Read the model definition and answer for the solid it produces. Units are mm, in the model's axes. Coordinates: 2 decimals unless noted, no trailing zeros. Order: outer loops, then holes, each group sorted by start corner. A loop starts at its lowest first (then second) coordinate and runs counter-clockwise, first axis right, second up.
Autodesk Inventor part; units mm, degrees
ref_plane "YZ Plane" through (0, 0, 0) normal (1, 0, 0) x (0, 1, 0)
ref_plane "XZ Plane" through (0, 0, 0) normal (0, 1, 0) x (-1, 0, 0)
ref_plane "XY Plane" through (0, 0, 0) normal (0, 0, 1) x (1, 0, 0)
sketch "Sketch1" plane through (0, 0, 0) normal (0, 1, 0) x (-1, 0, 0)
  line L0 (25.9, 0) -> (-25.9, 0)
  line L1 (0, -25.9) -> (0, 25.9)
  circle A0 centre (0, 0) radius 18.5 construction
  circle A1 centre (0, 0) radius 13 construction
  dimension "d0" = 37
  dimension "d1" = 26
sketch "Sketch2" plane through (0, 0, 0) normal (0, 1, 0) x (-1, 0, 0)
  line L0 (0, -28.9) -> (0, 26.4)
  line L1 (-60.5, -8) -> (-60.5, -21)
  line L2 (-60.5, -21) -> (60.5, -21)
  line L3 (60.5, -21) -> (60.5, -8)
  line L4 (60.5, -8) -> (-60.5, -8)
  line L5 (-84.7, 0) -> (84.7, 0)
  point P0 (0, 0)
  dimension "d3" = 121
  dimension "d99" = 8
  dimension "d101" = 21
extrude "Extrusion1" add sketch "Sketch2" along normal blind 6
sketch "Sketch6" plane through (0, 0, 0) normal (0, 1, 0) x (-1, 0, 0)
  line L0 (60.5, -21) -> (-60.5, -21)
  line L1 (60.5, -8) -> (60.5, -21)
  line L2 (-60.5, -21) -> (60.5, -21)
  line L3 (60.5, -21) -> (60.5, -8)
  line L4 (-60.5, -8) -> (-60.5, -21)
  line L5 (84.7, 0) -> (-84.7, 0)
  line L6 (0, -28.9) -> (0, 26.4)
  arc A0 (-16, 0) -> (16, 0) centre (0, 0) ccw
  line L7 (16, 0) -> (16, 0)
  line L8 (60.5, 0) -> (-60.5, 0)
  line L9 (16, 0) -> (60.5, 0)
  line L10 (-16, 0) -> (-16, 0)
  line L11 (-16, 0) -> (-60.5, 0)
  point P0 (-17.3617, -21)
  dimension "d18" = 32
extrude "Extrusion5" [suppressed]
sketch "Sketch4" plane through (0, 0, 0) normal (0, 0, 1) x (1, 0, 0)
  line L0 (-18.5, 0) -> (18.5, 0)
  line L1 (18.5, 0) -> (18.5, -2)
  line L2 (18.5, -2) -> (-18.5, -2)
  line L3 (-18.5, -2) -> (-18.5, 0)
  line L4 (-25.9, 0) -> (25.9, 0)
  line L5 (0, -2.4) -> (0, 0.4)
  point P0 (0, 0)
  dimension "d10" = 37
  dimension "d11" = 2
extrude "Extrusion6" [suppressed]
sketch "Sketch5" plane through (0, 0, 0) normal (0, 1, 0) x (-1, 0, 0)
  circle A0 centre (0, 0) radius 18.5 construction
  circle A1 centre (0, 0) radius 18.5 construction
  line L0 (25.9, 0) -> (-25.9, 0)
  line L1 (0, -28.9) -> (0, 26.4)
  line L2 (-18.5, -21) -> (18.5, -21)
  line L3 (18.5, -21) -> (18.5, -18.5)
  line L4 (18.5, -18.5) -> (-18.5, -18.5)
  line L5 (-18.5, -18.5) -> (-18.5, -21)
  dimension "d25" = 37
  dimension "d26" = 21
extrude "Extrusion7" [suppressed]
sketch "Sketch7" plane through (0, 0, 0) normal (0, 0, 1) x (1, 0, 0)
  line L0 (-18.5, 0) -> (18.5, 0)
  line L1 (18.5, 0) -> (18.5, -2)
  line L2 (18.5, -2) -> (-18.5, -2)
  line L3 (-18.5, -2) -> (-18.5, 0)
  line L4 (60.5, 0) -> (-60.5, 0)
  line L5 (-84.7, 0) -> (84.7, 0)
  line L6 (0, -2.4) -> (0, 0.4)
  point P0 (-16, 0)
  point P1 (16, 0)
  dimension "d53" = 2
  dimension "d54" = 18.5
extrude "Extrusion8" [suppressed]
sketch "Sketch8" plane through (0, 0, 0) normal (0, 1, 0) x (-1, 0, 0)
  circle A0 centre (0, 0) radius 12.75
  dimension "d34" = 25.5
extrude "Extrusion9" [suppressed]
pattern_linear "Rectangular Pattern1" [suppressed]
sketch "Sketch9" plane through (0, 6, 0) normal (0, 1, 0) x (1, 0, 0)
  circle A0 centre (0, 0) radius 13
  circle A1 centre (0, 0) radius 15
  dimension "d40" = 26
  dimension "d41" = 30
extrude "Extrusion10" [suppressed]
sketch "Sketch10" plane through (0, 5, 0) normal (0, 1, 0) x (1, 0, 0)
  arc A0 (16, 0) -> (-16, 0) centre (0, 0) ccw
  line L0 (1.5, -18) -> (-1.5, -18)
  line L1 (-29.4, 0) -> (29.4, 0)
  line L2 (0, 36.3) -> (0, -70.8)
  line L3 (1.5, -12) -> (-1.5, -12)
  line L4 (1.5, -12) -> (1.5, -18)
  line L5 (-1.5, -18) -> (-1.5, -12)
  dimension "d48" = 3
  dimension "d49" = 12
  dimension "d50" = 6
extrude "Extrusion11" [suppressed]
fillet "Fillet1" [suppressed]
sketch "Sketch11" plane through (0, 0, 0) normal (0, 1, 0) x (-1, 0, 0)
  line L0 (-60.5, -21) -> (60.5, -21)
  line L1 (60.5, -21) -> (60.5, -47)
  line L2 (60.5, -47) -> (-60.5, -47)
  line L3 (-60.5, -47) -> (-60.5, -21)
  line L4 (84.7, 0) -> (-84.7, 0)
  line L5 (0, -60.1) -> (0, 31.6)
  point P0 (0, 0)
  dimension "d57" = 26
  dimension "d58" = 21
  dimension "d59" = 121
extrude "Extrusion12" add sketch "Sketch11" along normal blind 6
sketch "Sketch12" plane through (0, 0, 0) normal (1, 0, 0) x (0, 1, 0)
  line L0 (6, -8) -> (6, -47)
  arc A0 (6, -16.5081) -> (5.7334, -47) centre (34, -32) ccw
  line L1 (-6.8, 0) -> (40.8, 0)
  line L2 (0, -66) -> (0, 67)
  line L3 (6, -16.5081) -> (6, -47)
  line L4 (6, -47) -> (5.7334, -47)
  line L5 (0, -47) -> (6, -47)
  point P0 (0, 0)
  point P1 (6, 48)
  dimension "d62" = 32
  dimension "d63" = 32
  dimension "d64" = 34
extrude "Extrusion13" cut sketch "Sketch12" along normal through all both and the other way through all
fillet "Fillet3" radius 8 1 edges at (0, 0, -47)
sketch "Sketch13" plane through (0, 0, 0) normal (0, 1, 0) x (-1, 0, 0)
  line L0 (84.7, 0) -> (-84.7, 0)
  line L1 (0, -57.9802) -> (0, 72.5866)
  line L2 (60.5, -8) -> (60.5, -39.3278)
  arc A0 (13.0815, 23.9185) -> (13.0815, 13.0815) centre (18.5, 18.5) ccw
  line L3 (-60.5, -8) -> (-60.5, -16.5081)
  arc A1 (-13.0815, 13.0815) -> (-13.0815, 23.9185) centre (-18.5, 18.5) ccw
  line L4 (18.5, 37) -> (18.5, 0)
  line L5 (-18.5, 0) -> (-18.5, 37)
  line L6 (18.5, 37) -> (18.5, -8)
  line L7 (-60.5, 0) -> (60.5, 0)
  line L8 (-18.5, -8) -> (-18.5, 37)
  arc A2 (-9.2871, 53) -> (-13.0815, 23.9185) centre (0, 37) ccw
  arc A3 (13.0815, 23.9185) -> (9.2871, 53) centre (0, 37) ccw
  arc A4 (-13.0815, 13.0815) -> (-18.5, 0) centre (0, 0) ccw
  arc A5 (18.5, 0) -> (13.0815, 13.0815) centre (0, 0) ccw
  point P0 (60.5, -39.3278)
  point P1 (-55.5, 48)
  point P2 (-60.5, -16.5081)
  dimension "d68" = 37
  dimension "d71" = 18.5
  dimension "d72" = 18.5
  dimension "d73" = 7.663
  dimension "d74" = 7.663
  dimension "d75" = 18.5
  dimension "d76" = 18.5
  dimension "d77" = 18.5
  dimension "d78" = 18.5
extrude "Extrusion14" [suppressed]
sketch "Sketch14" plane through (0, 0, 0) normal (0, 1, 0) x (-1, 0, 0)
  circle A0 centre (18.5, 18.5) radius 10
  line L0 (39.9, 0) -> (-39.9, 0)
  line L1 (0, -27.9) -> (0, 37.9)
  circle A1 centre (-18.5, 18.5) radius 10
  point P0 (0, 0)
  dimension "d84" = 18.5
  dimension "d85" = 18.5
  dimension "d86" = 20
  dimension "d89" = 37
extrude "Extrusion15" [suppressed]
fillet "Fillet4" [suppressed]
fillet "Fillet5" radius 8 2 edges at (-60.5, 3, -8) (60.5, 3, -8)
fillet "Fillet6" radius 5 5 edges at (58.1569, 6, -10.3431) (60.5, 6, -16.254) (-58.1569, 6, -10.3431) (-60.5, 6, -16.254) (0, 6, -8)
equation "\"d85\" = d84"
properties part number "NespressoSpeedfiller-6X-scraper"
1) A cutting plane is placed at A-A, the plane x = -30. Determine the outline of the cut face in (y, z), and give its area (3 significant figures).
A:
outline: (0, -39.33) arc R8 ccw to (5.73, -47) arc R32 cw to (6, -16.51) - (6, -13) arc R5 ccw to (1, -8) - (0, -8) - close
area: 133 mm2
2) A cutting plane is placed at B-B, the plane z = -35.5. Determine the outline of the cut face in (x, y), and give its area (3 significant figures).
A:
outline: (-60.5, 0) - (60.5, 0) - (60.5, 1) arc R5 ccw to (60.36, 2.19) - (-60.36, 2.19) arc R5 ccw to (-60.5, 1) - close
area: 265 mm2
3) Flat-ended cylindrical pins translate along their axes: pin 1 Ø6 at (x, z) = (32.5, -42.5) entering from +Y; pin 2 Ø2 at (x, z) = (13.5, -23.5) entering from +Y. Find the tip coordinate at first contact, or state that the pin passes through.
A:
pin 1: stops at y = 4.99
pin 2: stops at y = 3.44
4) Straight lines are drawn through the part: line 1 (Z direction, x = 52.5, y = 1); line 2 (Z direction, x = 16, y = 4.75); line 3 (X direction, y = 1.5, z = -33). For each, find the intervals that lie inside material, in ascending order.
A:
line 1: z = -43.2 to -8
line 2: z = -46.64 to -44.98, -19.02 to -9.69
line 3: x = -60.47 to 60.47
5) Determine the mould class of faces 1 (the flat face through (1, 6, -15)), 2 (the cylindrical face through (-1, 2, -32)), 3 (the cylindrical face through (-58.219, 0.507, -10.406)) for opening direction Z: pulls with the +Z half, pulls with the -Z half, needs draft (parallel to the pull), parting line crosses it, or undercut.
A:
face 1: needs draft
face 2: undercut
face 3: pulls with the +Z half
